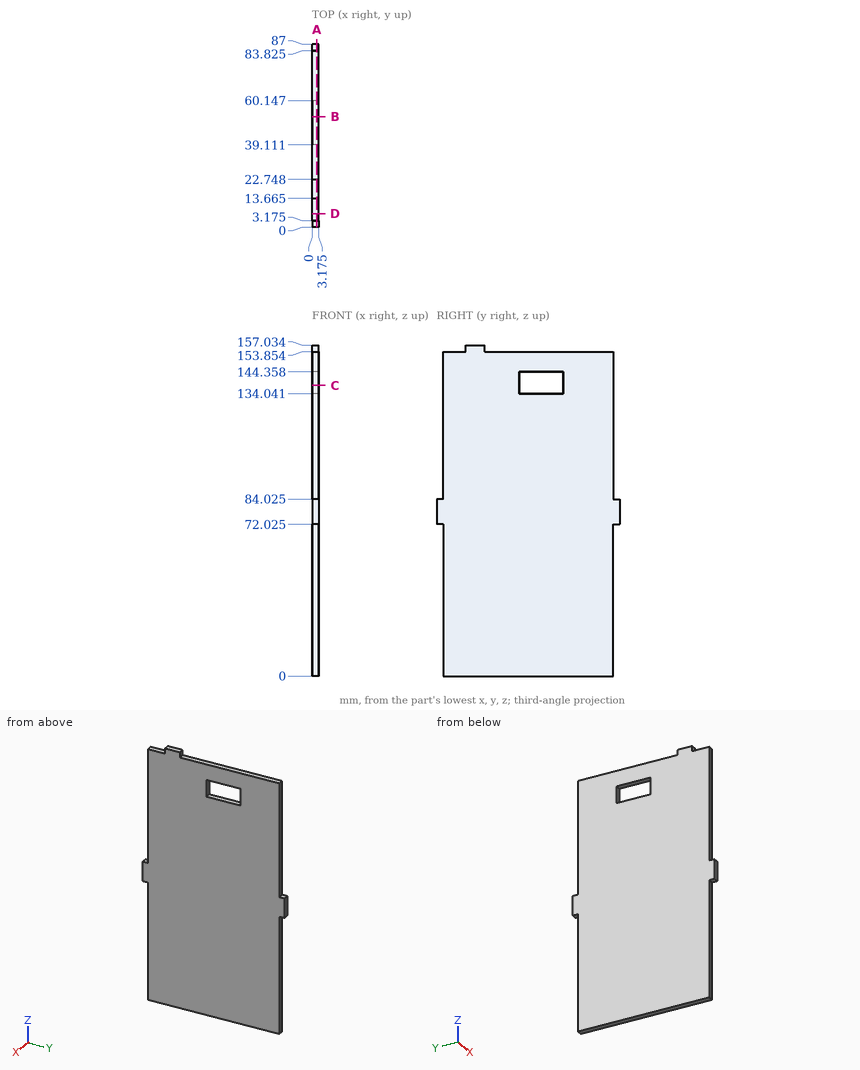
Drawing for the job (mm, zero at the part's lowest x, y, z). Give positions to 0.01 mm unless a question says otherwise; leave off trailing zeros. Loops run counter-clockwise (first coordinate to the right, second up) from the corner with the lowest first, then second, coordinate; pieces in that order, holes last. Notation, with made-up numbers: (26, 75.25) - (61, 75.25) arc R27 cw to (61, 107.25) - close; hole circle Ø11 at (68, 83). An arc over 180 degrees is marked (long way). Write item = value, one per line. Start each with the question number.
1) Band-saw the part on A-A on x = 2.25. Give the cut face in (y, z) (1 decimal).
2) Band-saw the part on B-B on y = 52.5. Give the cut face in (x, z) (1 decimal).
3) Band-saw the part on C-C on z = 138. Give the cut face in (x, y) (1 decimal), plus the area to 3 significant figures.
4) Drop flat-ended pins along their axis: pin 1 Ø1.6 at (x, y) = (1, 85.5) entering from +Z (3 decimals); pin 2 Ø1.6 at (x, z) = (1, 128.5) entering from +Y (3 decimals); pin 3 Ø1.6 at (x, y) = (1, 51) entering from +Z. Give the stop position or say it passes through.
5) Probe probe 1 along Z at (x, y) = (1.2, 49) (1 decimal); probe 2 along Y at (x, z) = (0.8, 44) (1 decimal); probe 3 along Z at (x, y) = (2.1, 82.5) (1 decimal). List the from-to ranges inside material, lowest first. Write a range as from..to.
6) Band-saw the part on D-D on y = 6.5. Give the cut face in (x, z) (1 decimal).
Final values:
q1.outline = (0, 72) - (3.2, 72) - (3.2, 0) - (83.8, 0) - (83.8, 72) - (87, 72) - (87, 84) - (83.8, 84) - (83.8, 153.9) - (22.7, 153.9) - (22.7, 157) - (13.7, 157) - (13.7, 153.9) - (3.2, 153.9) - (3.2, 84) - (0, 84) - close; hole (39.1, 134) - (60.1, 134) - (60.1, 144.4) - (39.1, 144.4) - close
q2.outline = (0, 0) - (3.2, 0) - (3.2, 134) - (0, 134) - close; (0, 144.4) - (3.2, 144.4) - (3.2, 153.9) - (0, 153.9) - close
q3.outline = (0, 3.2) - (3.2, 3.2) - (3.2, 39.1) - (0, 39.1) - close; (0, 60.1) - (3.2, 60.1) - (3.2, 83.8) - (0, 83.8) - close
q3.area = 189 mm²
q4.pin_1 = 84.025
q4.pin_2 = 83.825
q4.pin_3 = 153.85
q5.probe_1 = 0..134, 144.4..153.9
q5.probe_2 = 3.2..83.8
q5.probe_3 = 0..153.9
q6.outline = (0, 0) - (3.2, 0) - (3.2, 153.9) - (0, 153.9) - close
